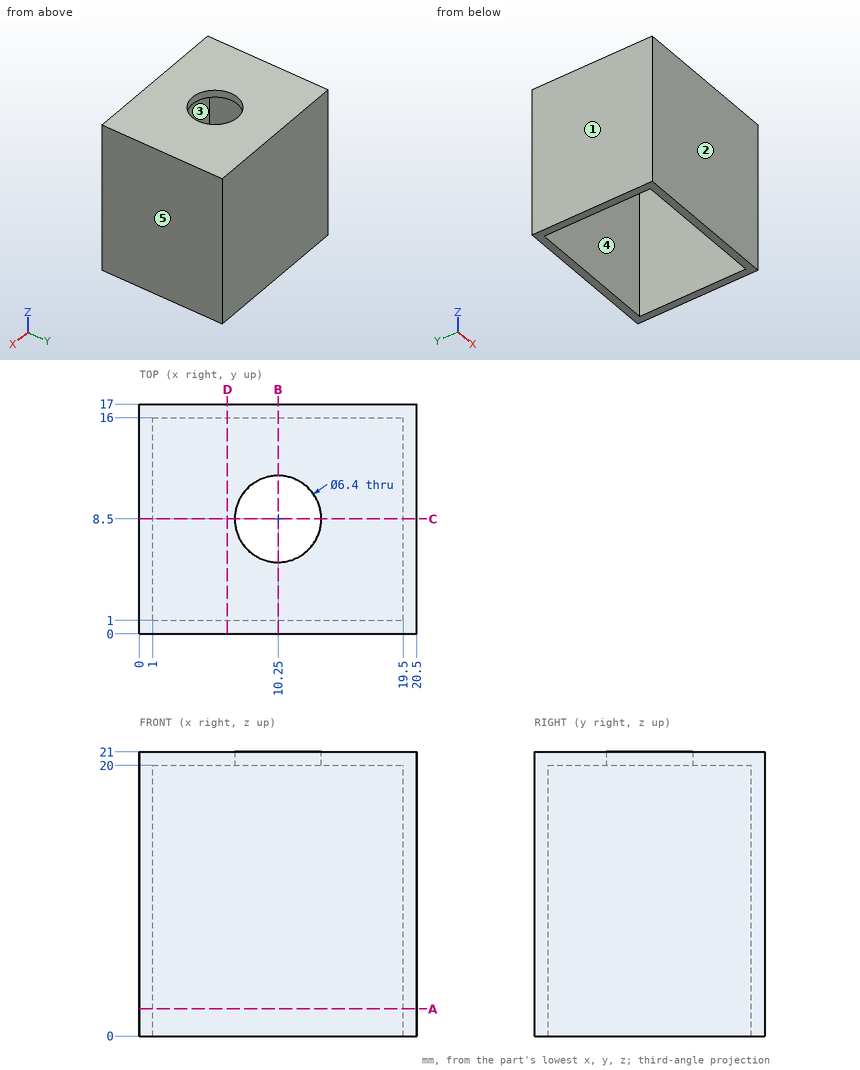
The figure shows three views and two pictorial views of one solid part (mm, origin at its lowest corner). Answer the questions. A direction names the side the tool comes from. Coordinates: 2 decimals unless noted, no trailing zeros. Loops run counter-clockwise (first coordinate to the right, second up) from the corner with the lowest first, then second, coordinate; pieces in that order, holes last. Notation, with made-up numbers: (-25.75, 36.5) -> (-17.75, 36.5) arc R15 ccw to (-17.75, 42.5) -> close; hole circle Ø1 at (-25.75, -33). An arc over 180 degrees is marked (long way). Return JSON: item names as keys, results as strings. Group by question number.
(1) Find the intervals of material crossed by probe 1 along Y at (x, z) = (10.25, 20.45); probe 2 along X at (y, z) = (2.75, 18.5); probe 3 along Y at (x, z) = (12, 12.75), in increasing order. Write a range as from..to.
(2) Which of the six approach directions +Z, -Z, +X, -X, +Y, -Y give full straight-line access (tool end or side, diameter ignored) to the marked faces 4 and 5?
(3) A cutting plane is placed at C-C on y = 8.5. Write down the section's boundary in (x, z), and give its area (3 significant figures).
(4) A cutting plane is placed at B-B on x = 10.25. Write down the section's boundary in (y, z).
(5) Determine the mould class of the marked faces 1, 2 and 3 for opening direction X: released by +X, released by -X, zero draft, split by the parting line, or undercut.
(6) A cutting plane is placed at D-D on x = 6.5. Write down the section's boundary in (y, z), and give its area (3 significant figures).
(7) A cutting plane is placed at A-A on z = 2. Write down the section's boundary in (x, y), and give its area (3 significant figures).
(8) Given pin 1 Ø8 at (x, y) = (12.5, 7.5) entering from -Z, flat-ended and moving along its own axis, determine where the tip first touches the part or whether it passes through.
The answers:
{
 "1": {"probe 1": "y = 0..5.3, 11.7..17", "probe 2": "x = 0..1, 19.5..20.5", "probe 3": "y = 0..1, 16..17"},
 "2": {"face 4": "-Z", "face 5": "+Z, -Z, +X, +Y, -Y"},
 "3": {"outline": "(0, 0) -> (1, 0) -> (1, 20) -> (7.05, 20) -> (7.05, 21) -> (0, 21) -> close; (13.45, 20) -> (19.5, 20) -> (19.5, 0) -> (20.5, 0) -> (20.5, 21) -> (13.45, 21) -> close", "area": "54.1 mm^2"},
 "4": {"outline": "(0, 0) -> (1, 0) -> (1, 20) -> (5.3, 20) -> (5.3, 21) -> (0, 21) -> close; (11.7, 20) -> (16, 20) -> (16, 0) -> (17, 0) -> (17, 21) -> (11.7, 21) -> close"},
 "5": {"face 1": "released by -X", "face 2": "zero draft", "face 3": "undercut"},
 "6": {"outline": "(0, 0) -> (1, 0) -> (1, 20) -> (16, 20) -> (16, 0) -> (17, 0) -> (17, 21) -> (0, 21) -> close", "area": "57.0 mm^2"},
 "7": {"outline": "(0, 0) -> (20.5, 0) -> (20.5, 17) -> (0, 17) -> close; hole (1, 1) -> (19.5, 1) -> (19.5, 16) -> (1, 16) -> close", "area": "71.0 mm^2"},
 "8": {"pin 1": "stops at z = 20"}
}
